```python
from build123d import *

# Parameters (mm, degrees)
SKETCH026_R  = 1.2
PAD023_DEPTH = 1.67
SKETCH027_R  = 2.5
SKETCH027_W  = 11.25
SKETCH027_H  = 11.25
PAD024_DEPTH = 1
FILLET005_R  = 0.5


with BuildPart() as part:
    # Sketch026 → Pad023 (new body)
    with BuildSketch(Plane.XY):
        Polygon((0.2, -0.2), (15, -0.2), (15, -10), (2.5, -10), (2.5, -22.5), (17.5, -22.5), (17.5, -31.412779), (47.5, -31.412779), (47.5, -2.5), (50, -2.5), (50, -0.2), (64.8, -0.2), (64.8, -7.5), (50, -7.5), (50, -31.412779), (57.5, -31.412779), (57.5, -22.5), (64.8, -22.5), (64.8, -32.3), (60, -32.3), (17.5, -32.3), (0.2, -32.3), (0.2, -22.5), (0.2, -10), align=None)
        with Locations((3.496368, -26.500834)):
            Circle(SKETCH026_R, mode=Mode.SUBTRACT)
        with Locations((3.486166, -3.492743)):
            Circle(SKETCH026_R, mode=Mode.SUBTRACT)
        with Locations((61.502525, -3.493081)):
            Circle(SKETCH026_R, mode=Mode.SUBTRACT)
        with Locations((61.5, -26.5)):
            Circle(SKETCH026_R, mode=Mode.SUBTRACT)
    extrude(amount=PAD023_DEPTH)

    # Sketch027 (on Face30 of Pad023) → Pad024 (join)
    with BuildSketch(Plane.XY.offset(1.67)):
        Polygon((-1.25, 1.25), (18.75, 1.25), (46.25, 1.25), (66.25, 1.25), (66.25, -11.25), (66.25, -18.75), (66.25, -33.75), (66.25, -38.75), (-1.25, -38.75), (-1.25, -33.75), (-1.25, -12.5), align=None)
        with Locations((61.25, -15)):
            Circle(SKETCH027_R, mode=Mode.SUBTRACT)
        with Locations((53.75, -21.25)):
            Circle(SKETCH027_R, mode=Mode.SUBTRACT)
        Polygon((18.75, 0), (18.75, -12.5), (18.75, -33.75), (46.25, -33.75), (46.25, -17.5), (46.25, -11.25), (46.25, 0), align=None, mode=Mode.SUBTRACT)
        with Locations((8.125, -16.875)):
            Rectangle(SKETCH027_W, SKETCH027_H, mode=Mode.SUBTRACT)
    extrude(amount=PAD024_DEPTH)

    # Fillet005
    fillet005_edges = [part.edges().sort_by_distance(p)[0] for p in [
        (-1.25, -5.625, 2.67),
        (8.75, 1.25, 2.67),
        (32.5, 1.25, 2.67),
        (56.25, 1.25, 2.67),
        (66.25, -5, 2.67),
        (66.25, -15, 2.67),
        (66.25, -26.25, 2.67),
        (66.25, -36.25, 2.67),
        (32.5, -38.75, 2.67),
        (-1.25, -36.25, 2.67),
        (-1.25, -23.125, 2.67),
        (18.75, -6.25, 2.67),
        (18.75, -23.125, 2.67),
        (32.5, -33.75, 2.67),
        (46.25, -25.625, 2.67),
        (46.25, -14.375, 2.67),
        (46.25, -5.625, 2.67),
        (32.5, 0, 2.67),
        (2.5, -16.875, 2.67),
        (8.125, -22.5, 2.67),
        (13.75, -16.875, 2.67),
        (8.125, -11.25, 2.67),
        (51.25, -21.25, 2.67),
        (58.75, -15, 2.67),
    ]]
    fillet(fillet005_edges, radius=FILLET005_R)


with BuildPart() as part_1:
    # Body004 placement: moved
    add(part.part.moved(Location((0, 0, 14))))


solid = part_1.part
```
Geometry: final body of the model. Coordinates: model frame, mm. A direction names the side the tool comes from. Round coordinates to 2 decimals unless told otherwise and drop trailing zeros. Order: outer loops, then holes, each group sorted by start corner. A loop starts at its lowest first (then second) coordinate and runs counter-clockwise, first axis right, second up. Notation, with made-up numbers: (72, -29) -> (83, -29) arc R23 cw to (83, 2) -> close; hole circle Ø5 at (35.5, -35.5). An arc over 180 degrees is marked (long way). Use one line per item in the form item = value.
(1) Section B-B on x = 21.5. Return loops of the section in (y, z).
Results list:
outline = (-38.75, 15.67) -> (-33.75, 15.67) -> (-33.75, 16.17) arc R0.5 ccw to (-34.25, 16.67) -> (-38.25, 16.67) arc R0.5 ccw to (-38.75, 16.17) -> close; (-32.3, 14) -> (-31.41, 14) -> (-31.41, 15.67) -> (-32.3, 15.67) -> close; (0, 15.67) -> (1.25, 15.67) -> (1.25, 16.17) arc R0.5 ccw to (0.75, 16.67) -> (0.5, 16.67) arc R0.5 ccw to (0, 16.17) -> close
(2) Section A-A on y = -28.5. Return loops of the section in (x, z).
Results list:
outline = (-1.25, 15.67) -> (0.2, 15.67) -> (0.2, 14) -> (17.5, 14) -> (17.5, 15.67) -> (18.75, 15.67) -> (18.75, 16.17) arc R0.5 ccw to (18.25, 16.67) -> (-0.75, 16.67) arc R0.5 ccw to (-1.25, 16.17) -> close; (46.25, 15.67) -> (47.5, 15.67) -> (47.5, 14) -> (50, 14) -> (50, 15.67) -> (57.5, 15.67) -> (57.5, 14) -> (64.8, 14) -> (64.8, 15.67) -> (66.25, 15.67) -> (66.25, 16.17) arc R0.5 ccw to (65.75, 16.67) -> (46.75, 16.67) arc R0.5 ccw to (46.25, 16.17) -> close
(3) Ray query, probe 1 along X at (y, z) = (-29.5, 14.75); probe 2 along Y at (x, z) = (6.5, 14.55); probe 3 along X at (y, z) = (-20, 14.2). Return the intervals inside material, ascending. Write a range as [from, to].
Results list:
probe_1 = [0.2, 17.5], [47.5, 50], [57.5, 64.8]
probe_2 = [-32.3, -22.5], [-10, -0.2]
probe_3 = [0.2, 2.5], [47.5, 50]
(4) Access query for faces 4 (the face through (62.61, -26.96, 14.82)), 5 (the face through (17.5, -27, 15)), 6 (the face through (32, -32.3, 15)), 7 (the face through (16, -23, 14)). Directions: +Z, -Z, +X, -X, +Y, -Y. A direction counts if a zero-diameter tool reaches every point of the face in a straight line with its end or side. Return the directions, or none.
Results list:
face_4 = -Z
face_5 = -Z, +Y
face_6 = -Z, +X, -X, -Y
face_7 = -Z, +X, -X, +Y, -Y
(5) Section C-C on y = -15. Count the separate pieces of the cut face and the enclosed holes in it, and give its area (3 significant figures).
Results list:
separate_pieces = 4
enclosed_holes = 0
area = 31.3 mm^2
(6) Draft query along X for faces 1 (the face through (56.135, -20.499, 15.916)), 2 (the face through (57, -0.2, 15)), 3 (the face through (64.8, -4, 15)). Return one class per face: pulls with the +X half, pulls with the -X half, needs draft (parallel to the pull), parting line crosses it, or undercut.
Results list:
face_1 = undercut
face_2 = needs draft
face_3 = pulls with the +X half
(7) First-contact query: pin 1 Ø0.8 at (x, z) = (48.5, 15) entering from +Y; pin 2 Ø2 at (x, y) = (3.5, -26.5) entering from -Z; pin 3 Ø0.8 at (y, z) = (-20, 14.5) entering from -X; pin 4 Ø3 at (x, y) = (61.25, -15) entering from -Z. Flat tips, straight axial feed; report the tip coordinate or a pass-through.
Results list:
pin_1 = -2.5
pin_2 = 15.67
pin_3 = 0.2
pin_4 = through
(8) Section D-D on x = 6. Return loops of the section in (y, z), and give its area (3 significant figures).
Results list:
outline = (-38.75, 15.67) -> (-32.3, 15.67) -> (-32.3, 14) -> (-22.5, 14) -> (-22.5, 16.17) arc R0.5 ccw to (-23, 16.67) -> (-38.25, 16.67) arc R0.5 ccw to (-38.75, 16.17) -> close; (-11.25, 15.67) -> (-10, 15.67) -> (-10, 14) -> (-0.2, 14) -> (-0.2, 15.67) -> (1.25, 15.67) -> (1.25, 16.17) arc R0.5 ccw to (0.75, 16.67) -> (-10.75, 16.67) arc R0.5 ccw to (-11.25, 16.17) -> close
area = 61.3 mm^2
